Input: part model. Units: mm. Frame: model coordinates. A direction names the side the tool comes from. Round coordinates to 2 decimals unless told otherwise and drop trailing zeros. Loops run counter-clockwise (first coordinate to the right, second up) from the corner with the lowest first, then second, coordinate; pieces in that order, holes last. Notation, with made-up numbers: (-15.75, 11.5) - (-10.75, 11.5) arc R12 ccw to (-10.75, 16.5) - close; hole circle Ø4 at (-13.75, -4.5). An arc over 180 degrees is marked (long way). One line per question, with ' | ' between items. Start each with the question number.
Item 1: First-contact query: pin 1 (12 mm diameter, centred on x = 14, y = -6.5, fed in from +Z); pin 2 (1.5 mm diameter, centred on x = -21.5, y = 17.5, fed in from +Z) (3 decimals); pin 3 (8.5 mm diameter, centred on x = 67, y = 10.5, fed in from -Z). Flat tips, straight axial feed; report the tip coordinate or a pass-through.
Item 2: Section B-B, the plane z = 6. Return loops of the section in (x, y) (3 decimals).
Item 3: Material intervals for line 1 along Z through (x, y) = (88.9, 9) (3 decimals); line 2 along Y through (x, z) = (5.5, 49); line 3 along Y through (x, z) = (66, 46), sorted ascending.
Item 4: Section A-A, the plane y = -22.5. Return loops of the section in (x, z) (3 decimals), plus the area to 3 significant figures.
Item 5: Set-up query: faces 1 (the face through (32.73, 16.55, 51.97)), 2 (the face through (45.8, -0.4, 38.1)), 3 (the face through (60, -2, 61.925)), 4 (the face through (22.225, -17, 18)), 5 (the face through (41.275, -1, 4)). Return all of +Z, -Z, +X, -X, +Y, -Y with unobstructed straight access to the full face (end or side cutting, diameter ignored); none if empty.
Item 6: Draft query along Z for faces 6 (the face through (60, 2, 42.875)), 7 (the face through (32.73, -16.79, 51.97)), 8 (the face through (22.225, 17, 18)), 9 (the face through (92.072, 0.356, 62.065)). Return one class per face: pulls with the +Z half, pulls with the -Z half, needs draft (parallel to the pull), parting line crosses it, or undercut.
Item 7: Section C-C, the plane x = 80.5. Return loops of the section in (y, z) (3 decimals).
```python
from build123d import *

# Parameters (mm, degrees)
F1_DEPTH = 63.5
F0_W     = 25.4
F0_H     = 19.05
F2_DEPTH = 25.4
F3_DEPTH = 7.9375
F5_R     = 6.35
F7_D     = 6.7564
F7_DEPTH = 12.7
F7_TIP   = 2.0298273432
F9_D     = 6.35


with BuildPart() as f1:
    # F0 (on Front) → F1 (new body, symmetric)
    with BuildSketch(Plane.XZ):
        Polygon((41.275, -9.525), (41.275, 9.525), (22.225, 9.525), (-41.275, 9.525), (-41.275, -9.525), align=None)
    extrude(amount=F1_DEPTH, both=True)

    # F0 (on Front) → F2 (join, symmetric)
    with BuildSketch(Plane.XZ):
        with BuildLine():
            Line((22.225, 9.525), (41.275, 9.525))
            Line((41.275, 9.525), (41.275, 27.0002))
            ThreePointArc((41.275, 27.0002), (45.9246798487, 38.2255201513), (57.15, 42.8752))
            Line((57.15, 42.8752), (60.325, 42.8752))
            Line((60.325, 42.8752), (60.325, 61.9252))
            Line((60.325, 61.9252), (57.15, 61.9252))
            ThreePointArc((57.15, 61.9252), (32.4542956671, 51.6959043329), (22.225, 27.0002))
            Line((22.225, 27.0002), (22.225, 9.525))
        make_face()
        with Locations((73.025, 52.4002)):
            Rectangle(F0_W, F0_H)
    extrude(amount=F2_DEPTH, both=True)

    # F0 (on Front) → F3 (join, symmetric)
    with BuildSketch(Plane.XZ):
        with BuildLine():
            Line((-41.275, 9.525), (22.225, 9.525))
            Line((22.225, 9.525), (22.225, 27.0002))
            ThreePointArc((22.225, 27.0002), (32.4542956671, 51.6959043329), (57.15, 61.9252))
            add(Edge.make_bspline(
                [(-41.275, 9.525), (-41.275, 34.8479822278), (9.3457987532, 61.9252), (57.15, 61.9252)],
                knots=[0, 0, 0, 0, 111.5045361635, 111.5045361635, 111.5045361635, 111.5045361635], degree=3))
        make_face()
    extrude(amount=F3_DEPTH, both=True)

    # F0 (on Front) → F4 (revolve)
    with BuildSketch(Plane.XZ):
        Polygon((85.725, 61.9252), (85.725, 42.8752), (85.725, 38.1), (111.125, 38.1), (111.125, 66.675), (85.725, 66.675), align=None)
    revolve(axis=Axis((85.725, 0, 52.3875), (0, 0, 1)))

    # F5
    f5_edges = [f1.edges().sort_by_distance(p)[0] for p in [
        (41.275, -63.5, 0),
        (-41.275, -63.5, 0),
        (41.275, 63.5, 0),
        (-41.275, 63.5, 0),
    ]]
    fillet(f5_edges, radius=F5_R)

    # F7
    with Locations(Plane.XY.offset(66.675)):
        with Locations((85.725, 0)):
            Hole(F7_D / 2, depth=F7_DEPTH)
            with Locations((0, 0, -(F7_DEPTH + F7_TIP / 2))):  # 118° drill point
                Cone(0, F7_D / 2, F7_TIP, mode=Mode.SUBTRACT)

    # F9 (through all)
    with Locations(Plane.XZ.offset(25.4)):
        with Locations((88.9, 61.9252)):
            Hole(F9_D / 2)


solid = f1.part
```
Return value:
1) pin 1: z = 56.88 | pin 2: z = 9.525 | pin 3: z = 38.1
2) outline: (-41.275, -57.15) arc R6.35 ccw to (-34.925, -63.5) - (34.925, -63.5) arc R6.35 ccw to (41.275, -57.15) - (41.275, 57.15) arc R6.35 ccw to (34.925, 63.5) - (-34.925, 63.5) arc R6.35 ccw to (-41.275, 57.15) - close
3) line 1: 38.1 to 58.75, 65.1 to 66.675 | line 2: -7.94 to 7.94 | line 3: -25.4 to 25.4
4) outline: (-41.275, -9.525) - (41.275, -9.525) - (41.275, 27) arc R15.875 cw to (57.15, 42.875) - (73.939, 42.875) - (73.939, 38.1) - (97.511, 38.1) - (97.511, 66.675) - (73.939, 66.675) - (73.939, 61.925) - (57.15, 61.925) arc R34.925 ccw to (22.225, 27) - (22.225, 9.525) - (-41.275, 9.525) - close; hole circle Ø6.35 at (88.9, 61.925) | area: 3,630 mm2
5) face 1: +Z, -X, +Y | face 2: -Z, +Y, -Y | face 3: +Z, -X | face 4: +Z, -X, -Y | face 5: -Z, +X, +Y, -Y
6) face 6: pulls with the -Z half | face 7: pulls with the +Z half | face 8: needs draft | face 9: undercut
7) outline: (-25.4, 42.875) - (-24.857, 42.875) - (-24.857, 38.1) - (24.857, 38.1) - (24.857, 42.875) - (25.4, 42.875) - (25.4, 61.925) - (24.857, 61.925) - (24.857, 66.675) - (-24.857, 66.675) - (-24.857, 61.925) - (-25.4, 61.925) - close
